Geometry: see drawing. Coordinates: mm, zero at the bounding-box minimum. Give positions to 0.01 mm unless a question says otherwise; leave off trailing zeros. Write each loop counter-clockwise with the first axis right and the second up, starting at its lowest first coordinate (ties: lowest second). Pieces come first, ordered by that corner, then holes. Notation, with made-up numbers: M 76.5,58.5 L 107.5,58.5 A23 ccw 107.5,71.5 Z; hole C -20,71 d4. An arc over 180 degrees is marked long. Use a Markdown table: item, result. Add a question column.
1) Section D-D on y = 132. Return the cut outline in (x, z) (1 decimal), then the cut area to 3 significant figures.
2) Section C-C on z = 61.5. Return the cut outline in (x, y) (1 decimal).
3) Section B-B on x = 4.25. State how many separate pieces and enclosed holes the cut face has, then the cut area to 3 significant figures.
4) Pin query (flat end, axial travel): pin 1 (6 mm diameter, centred on x = 8.5, z = 21.5, fed in from -Y); pin 2 (2 mm diameter, centred on x = 2, y = 122, fed in from +Z); pin 3 (5.5 mm diameter, centred on y = 200.04, z = 25.71, fed in from -X); pin 4 (10 mm diameter, centred on y = 200.04, z = 79.82, fed in from +X). Return the tip coordinate at first contact, or that it passes through.
5) Line query: line 1 (Z direction, x = 1, y = 200); line 2 (Y direction, x = 10.75, z = 39) (1 decimal); line 3 (Z direction, x = 1, y = 182). Output: solid intervals per line, ascending.
6) Section A-A on z = 39. Return the cut outline in (x, y) (1 decimal), then the cut area to 3 significant figures.
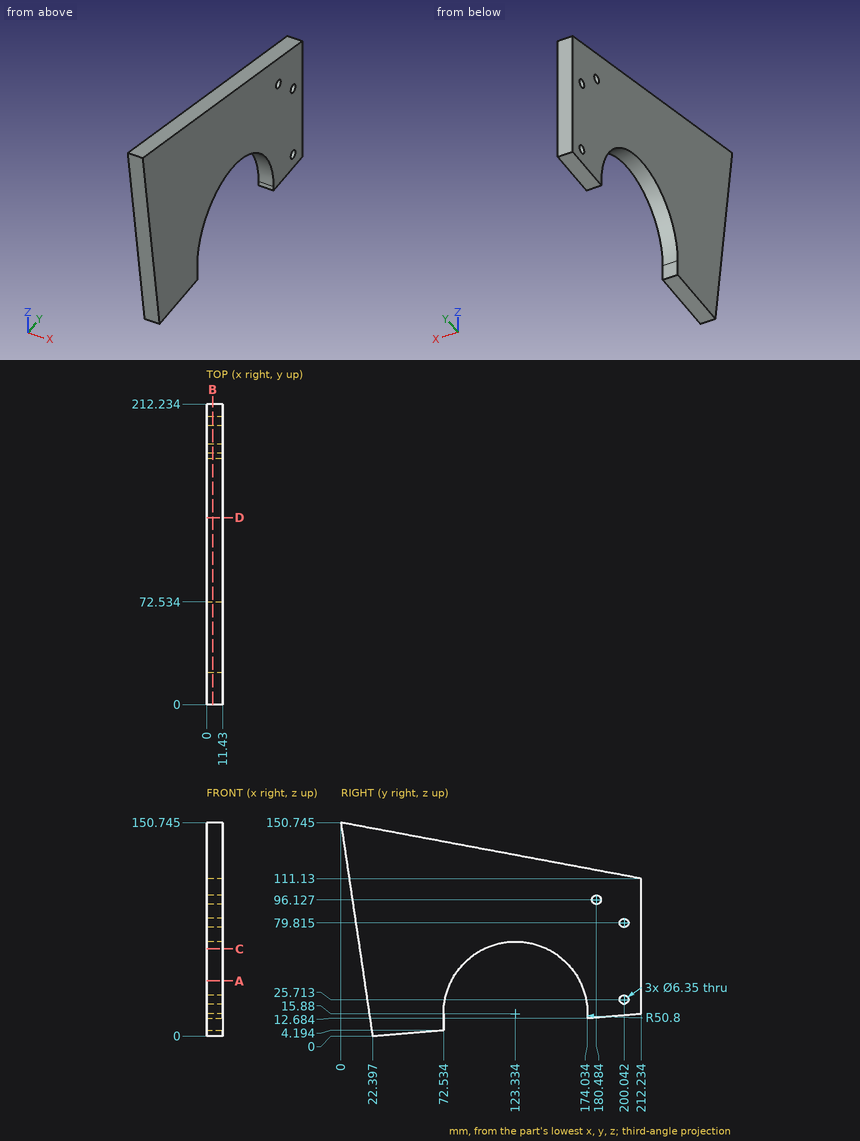
Found:
| question | item | result |
|---|---|---|
| 1 | outline | M 0,65.9 L 11.4,65.9 L 11.4,126.1 L 0,126.1 Z |
| 1 | area | 688 mm² |
| 2 | outline | M 0,13.3 L 11.4,13.3 L 11.4,101 L 0,101 Z; M 0,145.7 L 11.4,145.7 L 11.4,212.2 L 0,212.2 Z |
| 3 | separate pieces | 1 |
| 3 | enclosed holes | 3 |
| 3 | area | 19,700 mm² |
| 4 | pin 1 | y = 18.76 |
| 4 | pin 2 | z = 128.16 |
| 4 | pin 3 | through |
| 4 | pin 4 | x = 11.43 |
| 5 | line 1 | 14.86 to 22.54, 28.89 to 76.64, 82.99 to 113.41 |
| 5 | line 2 | 16.6 to 78.1, 168.6 to 212.2 |
| 5 | line 3 | 13.35 to 93.34, 98.92 to 116.77 |
| 6 | outline | M 0,16.6 L 11.4,16.6 L 11.4,78.1 L 0,78.1 Z; M 0,168.6 L 11.4,168.6 L 11.4,212.2 L 0,212.2 Z |
| 6 | area | 1,200 mm² |
